```python
from build123d import *

# Parameters (mm, degrees)
F0_R     = 26
F0_R_2   = 4.25
F1_DEPTH = 95


with BuildPart() as f1:
    # F0 (on Top) → F1 (new body)
    with BuildSketch(Plane.XY):
        Circle(F0_R)
        with BuildLine():
            ThreePointArc((1, 23.9791576166), (16.9705627485, 16.9705627485), (23.9791576166, 1))
            Line((23.9791576166, 1), (25, 1))
            Line((25, 1), (25, -1))
            Line((25, -1), (23.9791576166, -1))
            ThreePointArc((23.9791576166, -1), (16.9705627485, -16.9705627485), (1, -23.9791576166))
            Line((1, -23.9791576166), (1, -25))
            Line((1, -25), (-1, -25))
            Line((-1, -25), (-1, -23.9791576166))
            ThreePointArc((-1, -23.9791576166), (-16.9705627485, -16.9705627485), (-23.9791576166, -1))
            Line((-23.9791576166, -1), (-25, -1))
            Line((-25, -1), (-25, 1))
            Line((-25, 1), (-23.9791576166, 1))
            ThreePointArc((-23.9791576166, 1), (-16.9705627485, 16.9705627485), (-1, 23.9791576166))
            Line((-1, 23.9791576166), (-1, 25))
            Line((-1, 25), (1, 25))
            Line((1, 25), (1, 23.9791576166))
        make_face(mode=Mode.SUBTRACT)
        with BuildLine():
            ThreePointArc((-23.9791576166, -1), (-24, 0), (-23.9791576166, 1))
            Line((-23.9791576166, 1), (-25, 1))
            Line((-25, 1), (-25, -1))
            Line((-25, -1), (-23.9791576166, -1))
        make_face()
        with BuildLine():
            Line((1, -25), (1, -23.9791576166))
            ThreePointArc((1, -23.9791576166), (0, -24), (-1, -23.9791576166))
            Line((-1, -23.9791576166), (-1, -25))
            Line((-1, -25), (1, -25))
        make_face()
        with BuildLine():
            ThreePointArc((-1, -23.9791576166), (0, -24), (1, -23.9791576166))
            Line((1, -23.9791576166), (1, -6.1694813396))
            ThreePointArc((1, -6.1694813396), (0, -6.25), (-1, -6.1694813396))
            Line((-1, -6.1694813396), (-1, -23.9791576166))
        make_face()
        with BuildLine():
            Line((-6.1694813396, 1), (-23.9791576166, 1))
            ThreePointArc((-23.9791576166, 1), (-24, 0), (-23.9791576166, -1))
            Line((-23.9791576166, -1), (-6.1694813396, -1))
            ThreePointArc((-6.1694813396, -1), (-6.25, 0), (-6.1694813396, 1))
        make_face()
        with BuildLine():
            Line((-5, 1), (-6.1694813396, 1))
            ThreePointArc((-6.1694813396, 1), (-6.25, 0), (-6.1694813396, -1))
            Line((-6.1694813396, -1), (-5, -1))
            Line((-5, -1), (-5, 1))
        make_face()
        with BuildLine():
            ThreePointArc((23.9791576166, -1), (23.9947888384, -0.5001085894), (24, 0))
            ThreePointArc((24, 0), (23.9947888384, 0.5001085894), (23.9791576166, 1))
            Line((23.9791576166, 1), (6.1694813396, 1))
            ThreePointArc((6.1694813396, 1), (6.2298378138, 0.5016181951), (6.25, 0))
            ThreePointArc((6.25, 0), (6.2298378138, -0.5016181951), (6.1694813396, -1))
            Line((6.1694813396, -1), (23.9791576166, -1))
        make_face()
        with BuildLine():
            ThreePointArc((23.9791576166, 1), (23.9947888384, 0.5001085894), (24, 0))
            ThreePointArc((24, 0), (23.9947888384, -0.5001085894), (23.9791576166, -1))
            Line((23.9791576166, -1), (25, -1))
            Line((25, -1), (25, 1))
            Line((25, 1), (23.9791576166, 1))
        make_face()
        with BuildLine():
            Line((1, 6.1694813396), (1, 23.9791576166))
            ThreePointArc((1, 23.9791576166), (0, 24), (-1, 23.9791576166))
            Line((-1, 23.9791576166), (-1, 6.1694813396))
            ThreePointArc((-1, 6.1694813396), (0, 6.25), (1, 6.1694813396))
        make_face()
        with BuildLine():
            ThreePointArc((-1, 23.9791576166), (0, 24), (1, 23.9791576166))
            Line((1, 23.9791576166), (1, 25))
            Line((1, 25), (-1, 25))
            Line((-1, 25), (-1, 23.9791576166))
        make_face()
        with BuildLine():
            Line((1, 5), (1, 6.1694813396))
            ThreePointArc((1, 6.1694813396), (0, 6.25), (-1, 6.1694813396))
            Line((-1, 6.1694813396), (-1, 5))
            Line((-1, 5), (1, 5))
        make_face()
        with BuildLine():
            ThreePointArc((6.25, 0), (6.2298378138, 0.5016181951), (6.1694813396, 1))
            Line((6.1694813396, 1), (5, 1))
            Line((5, 1), (5, -1))
            Line((5, -1), (6.1694813396, -1))
            ThreePointArc((6.1694813396, -1), (6.2298378138, -0.5016181951), (6.25, 0))
        make_face()
        with BuildLine():
            Line((5, 1), (6.1694813396, 1))
            ThreePointArc((6.1694813396, 1), (4.4194173824, 4.4194173824), (1, 6.1694813396))
            Line((1, 6.1694813396), (1, 5))
            Line((1, 5), (-1, 5))
            Line((-1, 5), (-1, 6.1694813396))
            ThreePointArc((-1, 6.1694813396), (-4.4194173824, 4.4194173824), (-6.1694813396, 1))
            Line((-6.1694813396, 1), (-5, 1))
            Line((-5, 1), (-5, -1))
            Line((-5, -1), (-6.1694813396, -1))
            ThreePointArc((-6.1694813396, -1), (-4.4194173824, -4.4194173824), (-1, -6.1694813396))
            Line((-1, -6.1694813396), (-1, -5))
            Line((-1, -5), (1, -5))
            Line((1, -5), (1, -6.1694813396))
            ThreePointArc((1, -6.1694813396), (4.4194173824, -4.4194173824), (6.1694813396, -1))
            Line((6.1694813396, -1), (5, -1))
            Line((5, -1), (5, 1))
        make_face()
        Circle(F0_R_2, mode=Mode.SUBTRACT)
        with BuildLine():
            ThreePointArc((-1, -6.1694813396), (0, -6.25), (1, -6.1694813396))
            Line((1, -6.1694813396), (1, -5))
            Line((1, -5), (-1, -5))
            Line((-1, -5), (-1, -6.1694813396))
        make_face()
    extrude(amount=F1_DEPTH)


solid = f1.part
```
The listing builds one solid part. Answer for the finished solid, in the listing's coordinates (mm). A direction names the side the tool comes from. Give positions to 0.01 mm unless a question says otherwise; leave off trailing zeros. Write each loop counter-clockwise with the first axis right and the second up, starting at its lowest first coordinate (ties: lowest second). Pieces come first, ordered by that corner, then holes. Notation, with made-up numbers: M 41,3.25 L 97,3.25 A17 ccw 97,28.25 Z; hole C 68,-26.5 d2. An arc over 180 degrees is marked long. Write each question's results on one line, items separated by ' | '.
Q1. Flat-ended cylindrical pins translate along their axes: P1, Ø19.5, axis at x = 18.5, z = 71, coming from the +Y side; P2, Ø5, axis at x = -13.5, z = 83.5, coming from the -Y side; P3, Ø4, axis at x = 5.5, y = 5.5, coming from the +Z side; P4, Ø9, axis at x = -12, z = 49, coming from the +Y side. Find the tip coordinate at first contact, or state that the pin passes through.
Output values:
P1: y = 24.48 | P2: y = -23.56 | P3: z = 95 | P4: y = 24.89
Q2. Section A-A, the plane z = 31 is taken. Write down the section's boundary in (x, y), then the cut area to 3 significant figures.
Output values:
outline: C 0,0 d52; hole M -23.98,-1 A24 ccw -1,-23.98 L -1,-6.17 A6.25 cw -6.17,-1 Z; hole M -23.98,1 L -6.17,1 A6.25 cw -1,6.17 L -1,23.98 A24 ccw Z; hole C 0,0 d8.5; hole M 1,-23.98 A24 ccw 23.98,-1 L 6.17,-1 A6.25 cw 1,-6.17 Z; hole M 1,6.17 A6.25 cw 6.17,1 L 23.98,1 A24 ccw 1,23.98 Z | area: 522 mm2
Q3. A tool of negligible diameter and unlimited length cuts with its end or side. For faces 4 (the flat face through (-4, -2, 95)), 5 (the flat face through (-15, 1, 47)), from which of +Z, -Z, +X, -X, +Y, -Y can it reach the whole face along a straight path? Write none if from no direction.
Output values:
face 4: +Z, +X, -X, +Y, -Y | face 5: +Z, -Z
Q4. Section B-B, the plane y = 0 is taken. Write down the section's boundary in (x, z).
Output values:
outline: M -26,0 L -4.25,0 L -4.25,95 L -26,95 Z; M 4.25,0 L 26,0 L 26,95 L 4.25,95 Z
Q5. For a pull along X with two mould halves and no side action, classify faces 1 (the flat face through (15, 1, 47)), 2 (the flat face through (-4, -2, 0)), 3 (the cylindrical face through (-20.633, -15.821, 46.835)) as released by +X, released by -X, zero draft, split by the parting line, or undercut.
Output values:
face 1: undercut | face 2: zero draft | face 3: split by the parting line
Q6. Consider L1, parallel to X at y = 6.5, z = 89; L2, parallel to Y at x = -12, z = 71; L3, parallel to Y at x = 0, z = 33.5. Determine where each line is inside the solid, lowest interval first. Write a range as from..to.
Output values:
L1: -25.17..-23.1, -1..1, 23.1..25.17 | L2: -23.07..-20.78, -1..1, 20.78..23.07 | L3: -26..-4.25, 4.25..26
Q7. Section D-D, the plane y = 13.5 is taken. Write down the section's boundary in (x, z), then the cut area to 3 significant figures.
Output values:
outline: M -22.22,0 L -19.84,0 L -19.84,95 L -22.22,95 Z; M -1,0 L 1,0 L 1,95 L -1,95 Z; M 19.84,0 L 22.22,0 L 22.22,95 L 19.84,95 Z | area: 642 mm2
